Read the model definition and answer for the solid it produces. Units are mm, in the model's axes. A direction names the side the tool comes from. Round coordinates to 2 decimals unless told otherwise and drop trailing zeros. Loops run counter-clockwise (first coordinate to the right, second up) from the corner with the lowest first, then second, coordinate; pieces in that order, holes last. Notation, with made-up numbers: M 79.25,72.5 L 135.25,72.5 A27 cw 135.25,104.5 Z; hole C 79.5,32.5 d2. An arc over 180 degrees is marked long. Write each question's results on one line, items separated by ' | '.
```python
from build123d import *

# Parameters (mm, degrees)
SKETCH_1_W      = 40.7
SKETCH_1_H      = 42.9
EXTRUDE_1_DEPTH = 19.7
SKETCH_2_W      = 5
SKETCH_2_H      = 19.7
EXTRUDE_2_DEPTH = 10
SKETCH_3_R      = 9.85
EXTRUDE_3_DEPTH = 2
SKETCH_4_R      = 2.5
EXTRUDE_4_DEPTH = 5


with BuildPart() as part:
    # 草圖1 → 填料-伸長1 (new body)
    with BuildSketch(Plane.XY):
        with Locations((20.35, -21.45)):
            Rectangle(SKETCH_1_W, SKETCH_1_H)
    extrude(amount=EXTRUDE_1_DEPTH)

    # 草圖2 → 填料-伸長2 (add)
    with BuildSketch(Plane(origin=(0, 0, 0), x_dir=(1, 0, 0), z_dir=(0, 1, 0))):
        with Locations((7.5, -9.85)):
            Rectangle(SKETCH_2_W, SKETCH_2_H)
    extrude(amount=EXTRUDE_2_DEPTH)

    # 草圖3 → 填料-伸長3 (add)
    with BuildSketch(Plane.ZY):
        with Locations((9.85, -9.85)):
            Circle(SKETCH_3_R)
    extrude(amount=EXTRUDE_3_DEPTH)

    # 草圖4 → 填料-伸長4 (add)
    with BuildSketch(Plane.ZY.offset(2)):
        with Locations((9.85, -9.85)):
            Circle(SKETCH_4_R)
    extrude(amount=EXTRUDE_4_DEPTH)


solid = part.part
```
1. Find section D-D, the plane z = 1.75. Give the vertices of the cut face in (x, y).
Completed:
outline: M -2,-15.45 L 0,-15.45 L 0,-42.9 L 40.7,-42.9 L 40.7,0 L 10,0 L 10,10 L 5,10 L 5,0 L 0,0 L 0,-4.25 L -2,-4.25 Z
2. Given P1, Ø6, axis at y = -34.5, z = 15.5, coming from the -X side; P2, Ø6, axis at x = 30, z = 14, coming from the +Y side; P3, Ø8, axis at y = -3, z = 16, coming from the -X side, each flat-ended and moving along its own axis, determine where each tip first touches the part or whether it passes through.
Completed:
P1: stops at x = 0 | P2: stops at y = 0 | P3: stops at x = -2
3. Find section A-A, the plane z = 4.75. Give the vertices of the cut face in (x, y).
Completed:
outline: M -2,-18.28 L 0,-18.28 L 0,-42.9 L 40.7,-42.9 L 40.7,0 L 10,0 L 10,10 L 5,10 L 5,0 L 0,0 L 0,-1.42 L -2,-1.42 Z
4. Find section B-B, the plane y = -16. Give the vertices of the cut face in (x, z), then the cut area to 3 significant figures.
Completed:
outline: M -2,2.16 L 0,2.16 L 0,0 L 40.7,0 L 40.7,19.7 L 0,19.7 L 0,17.54 L -2,17.54 Z | area: 833 mm2
5. Find the intervals of material crossed by L1, parallel to Y at x = 20, z = 15; L2, parallel to X at y = -39.5, z = 1.25; L3, parallel to X at y = 4.5, z = 5.5, in increasing order.
Completed:
L1: y = -42.9 to 0 | L2: x = 0 to 40.7 | L3: x = 5 to 10
6. Find section C-C, the plane x = 32. Give the vertices of the cut face in (y, z), then the cut area to 3 significant figures.
Completed:
outline: M -42.9,0 L 0,0 L 0,19.7 L -42.9,19.7 Z | area: 845 mm2
7. Which of the six approach directions +Z, -Z, +X, -X, +Y, -Y give full straight-line access (tool end or side, diameter ignored) to faces 1 (the face through (0, -2, 2)), 2 (the face through (-0.986, -3.193, 2.59)), 3 (the face through (10, 5, 10)), 4 (the face through (2, 0, 10)), 5 (the face through (0, -2, 18))?
Completed:
face 1: -Z, -X, +Y | face 2: -X | face 3: +Z, -Z, +X, +Y | face 4: +Z, -Z, -X, +Y | face 5: +Z, -X, +Y
